Autodesk Inventor part; units mm, degrees
ref_plane "Work Plane1" through (10, 10, 0) normal (0, 1, 0) x (1, 0, 0)
ref_plane "YZ Plane" through (0, 0, 0) normal (1, 0, 0) x (0, 1, 0)
ref_plane "XZ Plane" through (0, 0, 0) normal (0, 1, 0) x (-1, 0, 0)
sketch "Sketch1" plane through (0, 0, 0) normal (0, 0, 1) x (1, 0, 0)
  line L0 (0, 0) -> (20, 0)
  line L1 (20, 0) -> (20, 20)
  line L2 (20, 20) -> (0, 20)
  line L3 (0, 20) -> (0, 0)
  line L4 (-10, 5) -> (30, 5)
  line L5 (30, 5) -> (30, 15)
  line L6 (30, 15) -> (-10, 15)
  line L7 (-10, 15) -> (-10, 5)
  line L8 (-10, 5) -> (30, 15) construction
  line L9 (30, 5) -> (-10, 15) construction
  circle A0 centre (10, 10) radius 4.05
  point P0 (20, 5)
  point P1 (20, 15)
  dimension "d0" = 20
  dimension "d1" = 20
  dimension "d2" = 40
  dimension "d3" = 10
  dimension "d4" = 10
  dimension "d5" = 10
  dimension "d6" = 8.1
extrude "Extrusion1" add sketch "Sketch1" along normal blind 26 contours L3 L4 L1 L0 | L3 L6 L1 L4 | L1 L6 L5 L4 | L3 L2 L1 L6
chamfer "Chamfer1" distance 2 angle 45 6 edges at (20, 20, 13) (30, 15, 13) (30, 5, 13) (20, 0, 13) (0, 20, 13) (0, 0, 13)
extrude "Extrusion2" add sketch "Sketch1" along normal blind 10 contours A0
fillet "Fillet2" radius 1 1 edges at (5.95, 10, 26)
ref_plane "Work Plane1" through (10, 10, 0) normal (0, 1, 0) x (1, 0, 0)
sketch "Sketch2" plane through (10, 10, 0) normal (0, 1, 0) x (1, 0, 0)
  line L0 (-10, 0) -> (-210, 0)
  line L1 (-210, 0) -> (-210, -3)
  line L2 (-210, -3) -> (-30, -3)
  line L3 (-10, 0) -> (-10, -26)
  line L4 (-10, -23) -> (-10, -26)
  arc A0 (-10, -23) -> (-30, -3) centre (-30, -23) ccw
  point P0 (-10, -3)
  dimension "d16" = 200
  dimension "d17" = 3
  dimension "d18" = 200
  dimension "d19" = 90
  dimension "d20" = 20
extrude "Extrusion3" add sketch "Sketch2" along normal mid plane 10
fillet "Fillet3" radius 1 6 edges at (-100, 5, 0) (-100, 15, 0) (-5.8579, 5, 8.8579) (-110, 5, 3) (-5.8579, 15, 8.8579) (-110, 15, 3)
properties part number "Turret_Holder_2_test"
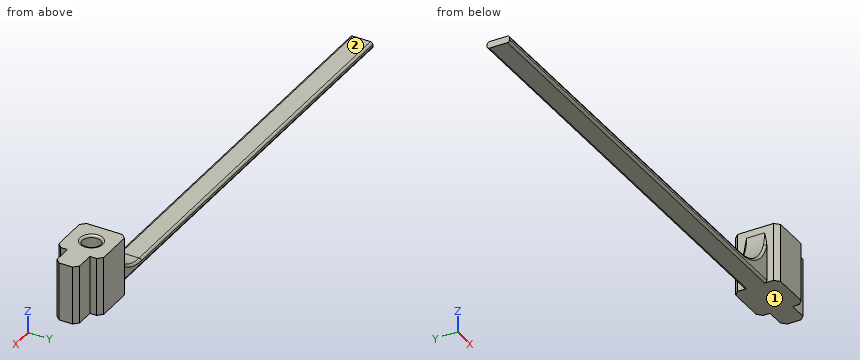
Verification items for the finished model (mm, model axes). Face numbers are marked on the shaded views. A direction names the side the tool comes from. Coordinates: 2 decimals unless noted, no trailing zeros. Loops run counter-clockwise (first coordinate to the right, second up) from the corner with the lowest first, then second, coordinate; pieces in that order, holes last. Notation, with made-up numbers: (4.5, 67.25) -> (42.5, 67.25) arc R17 cw to (42.5, 75.25) -> close; hole circle Ø4 at (-22, -28). An arc over 180 degrees is marked (long way). Put each result on its own line as item: value.
1. Section check A-A, the plane x = -77. Record the boundary of the cut face in (y, z).
Result set:
outline: (5, 1) arc R1 ccw to (6, 0) -> (14, 0) arc R1 ccw to (15, 1) -> (15, 2) arc R1 ccw to (14, 3) -> (6, 3) arc R1 ccw to (5, 2) -> close
2. Gauge pin test, flat ends, axial feed: P1, Ø10, axis at y = 9.5, z = 22.5, coming from the -X side; P2, Ø1, axis at x = -160.5, y = 9, coming from the +Z side; P3, Ø2.5, axis at x = 23.5, z = 7, coming from the +Y side; P4, Ø2, axis at x = -40, y = 17, coming from the -Z side. Record the tip position at first contact, or that the pin passes through.
Result set:
P1: stops at x = -0.77
P2: stops at z = 3
P3: stops at y = 15
P4: passes through
3. Thickness scan on line 1 (Y direction, x = 10, z = 15.5); line 2 (Y direction, x = -94.5, z = 1.75); line 3 (X direction, y = 17.25, z = 2.75). Record the ranges inside material, lowest first.
Result set:
line 1: y = 0 to 5.95, 14.05 to 20
line 2: y = 5 to 15
line 3: x = 0 to 20
4. Section check C-C, the plane x = 10. Record the boundary of the cut face in (y, z).
Result set:
outline: (0, 0) -> (20, 0) -> (20, 26) -> (15.05, 26) arc R1 ccw to (14.05, 25) -> (14.05, 10) -> (5.95, 10) -> (5.95, 25) arc R1 ccw to (4.95, 26) -> (0, 26) -> close
5. Tool access check on the marked faces 1 and 2. Record the directions out of +Z, -Z, +X, -X, +Y, -Y that give a thin tool (end or side, any length) a straight path to the whole face; none if there is none.
Result set:
face 1: -Z, +X, -X, +Y, -Y
face 2: +Z, -X, +Y, -Y
6. Section check B-B, the plane y = 10. Record the boundary of the cut face in (x, z), then the cut area to 3 significant figures.
Result set:
outline: (-200, 0) -> (30, 0) -> (30, 26) -> (15.05, 26) arc R1 ccw to (14.05, 25) -> (14.05, 10) -> (5.95, 10) -> (5.95, 25) arc R1 ccw to (4.95, 26) -> (0, 26) -> (0, 23) arc R20 cw to (-20, 3) -> (-200, 3) -> close
area: 1,340 mm^2
